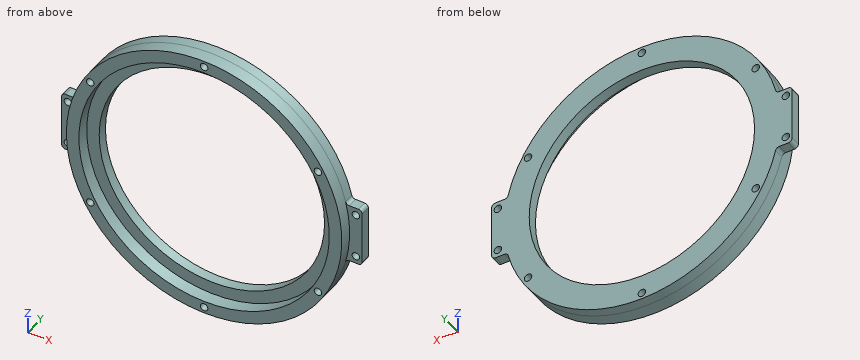
from build123d import *

# Parameters (mm, degrees)
SKETCH_1_R      = 1.5
SKETCH_1_R_2    = 45
EXTRUDE_1_DEPTH = 4
EXTRUDE_START   = -5
SKETCH_2_R      = 55
SKETCH_2_R_2    = 1.5
SKETCH_2_R_3    = 50
EXTRUDE_2_DEPTH = 5


with BuildPart() as part:
    # 草图1 → 凸台-拉伸1 (new body)
    with BuildSketch(Plane(origin=(0, 0, 0), x_dir=(1, 0, 0), z_dir=(0, 1, 0))):
        with BuildLine():
            ThreePointArc((-54.863466897, 12), (-53.938159008, 12.31940468), (-53.406914679, 13.14159292))
            ThreePointArc((-53.406914679, 13.14159292), (0, 55), (53.406914679, 13.14159292))
            ThreePointArc((53.406914679, 13.14159292), (53.938159008, 12.31940468), (54.863466897, 12))
            Line((54.863466897, 12), (58.5, 12))
            ThreePointArc((58.5, 12), (59.560660172, 11.560660172), (60, 10.5))
            Line((60, 10.5), (60, -10.5))
            ThreePointArc((60, -10.5), (59.560660172, -11.560660172), (58.5, -12))
            Line((58.5, -12), (54.863466897, -12))
            ThreePointArc((54.863466897, -12), (53.938159008, -12.31940468), (53.406914679, -13.14159292))
            ThreePointArc((53.406914679, -13.14159292), (0, -55), (-53.406914679, -13.14159292))
            ThreePointArc((-53.406914679, -13.14159292), (-53.938159008, -12.31940468), (-54.863466897, -12))
            Line((-54.863466897, -12), (-58.5, -12))
            ThreePointArc((-58.5, -12), (-59.560660172, -11.560660172), (-60, -10.5))
            Line((-60, -10.5), (-60, 10.5))
            ThreePointArc((-60, 10.5), (-59.560660172, 11.560660172), (-58.5, 12))
            Line((-58.5, 12), (-54.863466897, 12))
        make_face()
        with Locations(Location((-45.466333699, 26.25, 0), (0, 0, 270))):
            Circle(SKETCH_1_R, mode=Mode.SUBTRACT)
        with Locations(Location((-45.466333699, -26.25, 0), (0, 0, 270))):
            Circle(SKETCH_1_R, mode=Mode.SUBTRACT)
        with Locations(Location((0, -52.5, 0), (0, 0, 270))):
            Circle(SKETCH_1_R, mode=Mode.SUBTRACT)
        with Locations(Location((45.466333699, -26.25, 0), (0, 0, 270))):
            Circle(SKETCH_1_R, mode=Mode.SUBTRACT)
        with Locations(Location((45.466333699, 26.25, 0), (0, 0, 270))):
            Circle(SKETCH_1_R, mode=Mode.SUBTRACT)
        with Locations(Location((0, 52.5, 0), (0, 0, 270))):
            Circle(SKETCH_1_R, mode=Mode.SUBTRACT)
        with Locations(Location((57.5, 9, 0), (0, 0, 270))):
            Circle(SKETCH_1_R, mode=Mode.SUBTRACT)
        with Locations(Location((-57.5, -9, 0), (0, 0, 270))):
            Circle(SKETCH_1_R, mode=Mode.SUBTRACT)
        with Locations(Location((-57.5, 9, 0), (0, 0, 270))):
            Circle(SKETCH_1_R, mode=Mode.SUBTRACT)
        with Locations(Location((0, 0, 0), (0, 0, 270))):
            Circle(SKETCH_1_R_2, mode=Mode.SUBTRACT)
        with Locations(Location((57.5, -9, 0), (0, 0, 270))):
            Circle(SKETCH_1_R, mode=Mode.SUBTRACT)
    extrude(amount=EXTRUDE_1_DEPTH)

    # 草图2 → 凸台-拉伸2 (add)
    with BuildSketch(Plane(origin=(0, 0, 0), x_dir=(1, 0, 0), z_dir=(0, 1, 0)).offset(EXTRUDE_START)):
        with Locations(Location((0, 0, 0), (0, 0, 13.823871882))):
            Circle(SKETCH_2_R)
        with Locations(Location((-45.466333699, 26.25, 0), (0, 0, 270))):
            Circle(SKETCH_2_R_2, mode=Mode.SUBTRACT)
        with Locations(Location((-45.466333699, -26.25, 0), (0, 0, 270))):
            Circle(SKETCH_2_R_2, mode=Mode.SUBTRACT)
        with Locations(Location((0, -52.5, 0), (0, 0, 270))):
            Circle(SKETCH_2_R_2, mode=Mode.SUBTRACT)
        with Locations(Location((45.466333699, -26.25, 0), (0, 0, 270))):
            Circle(SKETCH_2_R_2, mode=Mode.SUBTRACT)
        with Locations(Location((45.466333699, 26.25, 0), (0, 0, 270))):
            Circle(SKETCH_2_R_2, mode=Mode.SUBTRACT)
        with Locations(Location((0, 52.5, 0), (0, 0, 270))):
            Circle(SKETCH_2_R_2, mode=Mode.SUBTRACT)
        with Locations(Location((0, 0, 0), (0, 0, 270))):
            Circle(SKETCH_2_R_3, mode=Mode.SUBTRACT)
    extrude(amount=EXTRUDE_2_DEPTH)


solid = part.part
Work out the finished part from the listing and answer in its coordinate system (mm). Give positions to 0.01 mm unless a question says otherwise; leave off trailing zeros. Write each loop counter-clockwise with the first axis right and the second up, starting at its lowest first coordinate (ties: lowest second). Pieces come first, ordered by that corner, then holes.
Q1. The part is cut by section A-A on z = 0. Give the vertices of the cut face in (x, y).
Answer:
outline: (-60, 0) - (-55, 0) - (-55, -5) - (-50, -5) - (-50, 0) - (-45, 0) - (-45, 4) - (-60, 4) - close; (45, 0) - (50, 0) - (50, -5) - (55, -5) - (55, 0) - (60, 0) - (60, 4) - (45, 4) - close
Q2. The part is cut by section B-B on x = -24. Give the vertices of the cut face in (y, z), and give its area (3 significant figures).
Answer:
outline: (-5, -49.49) - (4, -49.49) - (4, -38.07) - (0, -38.07) - (0, -43.86) - (-5, -43.86) - close; (-5, 43.86) - (0, 43.86) - (0, 38.07) - (4, 38.07) - (4, 49.49) - (-5, 49.49) - close
area: 148 mm2
Q3. Given pin 1 (1.1 mm diameter, centred on x = 57, y = 2, fed in from +Z); pin 2 (3.5 mm diameter, centred on x = 57.5, z = -1, fed in from -Y); pin 3 (2.5 mm diameter, centred on x = 45.47, z = -26.25, fed in from -Y); pin 4 (1.5 mm diameter, centred on y = 0.5, z = -20, fed in from +X), each flat-ended and moving along its own axis, determine where each tip first touches the part or whether it passes through.
Answer:
pin 1: stops at z = 12
pin 2: stops at y = 0
pin 3: passes through
pin 4: stops at x = 51.52
Q4. The part is cut by section C-C on y = -3.25. Give the vertices of the cut face in (x, z), and give its area (3 significant figures).
Answer:
outline: circle Ø110 at (0, 0); hole circle Ø100 at (0, 0); hole circle Ø3 at (-45.47, -26.25); hole circle Ø3 at (-45.47, 26.25); hole circle Ø3 at (0, -52.5); hole circle Ø3 at (0, 52.5); hole circle Ø3 at (45.47, -26.25); hole circle Ø3 at (45.47, 26.25)
area: 1,610 mm2
Q5. The part is cut by section D-D on x = 23. Give the vertices of the cut face in (y, z), and give its area (3 significant figures).
Answer:
outline: (-5, -49.96) - (4, -49.96) - (4, -38.68) - (0, -38.68) - (0, -44.4) - (-5, -44.4) - close; (-5, 44.4) - (0, 44.4) - (0, 38.68) - (4, 38.68) - (4, 49.96) - (-5, 49.96) - close
area: 146 mm2
Q6. Straight lines are drawn through the part: L1, parallel to X at y = 2.95, z = 9; L2, parallel to X at y = 1.45, z = 0; L3, parallel to X at y = 0.25, z = -26.5. For each, find the intervals that lie inside material, in ascending order.
Answer:
L1: x = -60 to -59, -56 to -44.09, 44.09 to 56, 59 to 60
L2: x = -60 to -45, 45 to 60
L3: x = -48.19 to -46.95, -43.99 to -36.37, 36.37 to 43.99, 46.95 to 48.19
